```python
from build123d import *

# Parameters (mm, degrees)
SKETCH3_W              = 20
SKETCH3_H              = 50
BOSS_EXTRUDE1_DEPTH    = 35
SKETCH4_R              = 4.75
CUT_EXTRUDE1_DEPTH     = 60
SKETCH5_R              = 3
CUT_EXTRUDE2_DEPTH     = 60
EXTRUDE_2_DEPTH        = 20
SKETCH_3_R             = 2
EXTRUDE_4_DEPTH        = 5
PATTERN_LINEAR_1_COUNT = 2
PATTERN_LINEAR_1_PITCH = 15
SKETCH_5_W             = 20
SKETCH_5_H             = 50
EXTRUDE_5_DEPTH        = 15
SKETCH_6_W             = 4.961104437
SKETCH_6_H             = 10
CUT_EXTRUDE_1_DEPTH    = 10
SKETCH_7_R             = 1.5
CUT_EXTRUDE_2_DEPTH    = 20
SKETCH_8_R             = 4
CUT_EXTRUDE_3_DEPTH    = 20
FILLET_11_R            = 5
FILLET_12_R            = 5
FILLET_START           = -0.209677419
FILLET_13_DEPTH        = 30


with BuildPart() as part:
    # Sketch3 → Boss-Extrude1 (new body)
    with BuildSketch(Plane(origin=(0, 0, 0), x_dir=(1, 0, 0), z_dir=(0, 1, 0))):
        with Locations((-3.806451613, -14.790322581)):
            Rectangle(SKETCH3_W, SKETCH3_H)
    extrude(amount=BOSS_EXTRUDE1_DEPTH)

    # Sketch4 → Cut-Extrude1 (cut)
    with BuildSketch(Plane.XY.offset(39.790322581)):
        with Locations((-3.806451613, 10)):
            Circle(SKETCH4_R)
    extrude(amount=-CUT_EXTRUDE1_DEPTH, mode=Mode.SUBTRACT)

    # Sketch5 → Cut-Extrude2 (cut)
    with BuildSketch(Plane(origin=(6.193548387, 0, 0), x_dir=(0, 0, -1), z_dir=(1, 0, 0))):
        with Locations((-34.790322581, 25)):
            Circle(SKETCH5_R)
        with Locations((5.209677419, 25)):
            Circle(SKETCH5_R)
    extrude(amount=-CUT_EXTRUDE2_DEPTH, mode=Mode.SUBTRACT)

    # 草圖2 → 填料-伸長2 (add)
    with BuildSketch(Plane(origin=(6.193548387, 0, 0), x_dir=(0, 0, -1), z_dir=(1, 0, 0))):
        Polygon((10.209677419, 32.525099494), (10.209677419, 17.525099494), (13.209677419, 22.525099494), (13.209677419, 27.525099494), align=None)
        Polygon((-39.790322581, 17.525099494), (-42.790322581, 22.525099494), (-42.790322581, 27.525099494), (-39.790322581, 32.525099494), align=None)
    extrude(amount=-EXTRUDE_2_DEPTH)

    # 草圖3 → 填料-伸長4 (add)
    # profile 1 of 2: a face of its own
    with BuildSketch(Plane(origin=(6.193548387, 0, 0), x_dir=(0, 0, -1), z_dir=(1, 0, 0))):
        with BuildLine():
            Line((13.209677419, 27.525099494), (17.601982265, 24.989201109))
            ThreePointArc((17.601982265, 24.989201109), (19.46568557, 20.489823314), (15.601982265, 17.525099494))
            Line((15.601982265, 17.525099494), (10.209677419, 17.525099494))
            Line((10.209677419, 17.525099494), (13.209677419, 22.525099494))
            Line((13.209677419, 22.525099494), (13.209677419, 27.525099494))
        make_face()
        with Locations((15.601982265, 21.525099494)):
            Circle(SKETCH_3_R, mode=Mode.SUBTRACT)
    # profile 2 of 2: a face of its own
    with BuildSketch(Plane(origin=(6.193548387, 0, 0), x_dir=(0, 0, -1), z_dir=(1, 0, 0))):
        with BuildLine():
            Line((-39.790322581, 17.525099494), (-45.182627426, 17.525099494))
            ThreePointArc((-45.182627426, 17.525099494), (-49.046330731, 20.489823314), (-47.182627426, 24.989201109))
            Line((-47.182627426, 24.989201109), (-42.790322581, 27.525099494))
            Line((-42.790322581, 27.525099494), (-42.790322581, 22.525099494))
            Line((-42.790322581, 22.525099494), (-39.790322581, 17.525099494))
        make_face()
        with Locations(Location((-45.182627426, 21.525099494, 0), (0, 0, 180))):
            Circle(SKETCH_3_R, mode=Mode.SUBTRACT)
    extrude_4 = extrude(amount=-EXTRUDE_4_DEPTH)

    # 直線複製排列1: 填料-伸長4 ×2
    with Locations(*[(-i * PATTERN_LINEAR_1_PITCH, 0, 0) for i in range(1, PATTERN_LINEAR_1_COUNT)]):
        add(extrude_4)

    # 草圖5 → 填料-伸長5 (add)
    with BuildSketch(Plane(origin=(0, 35, 0), x_dir=(1, 0, 0), z_dir=(0, 1, 0))):
        with Locations((-23.806451613, -14.790322581)):
            Rectangle(SKETCH_5_W, SKETCH_5_H)
    extrude(amount=-EXTRUDE_5_DEPTH)

    # 草圖6 → 除料-伸長1 (cut)
    with BuildSketch(Plane.XZ.offset(-20)):
        with Locations((-16.287003832, -5.209677419)):
            Rectangle(SKETCH_6_W, SKETCH_6_H)
        with Locations((-16.287003832, 34.790322581)):
            Rectangle(SKETCH_6_W, SKETCH_6_H)
    extrude(amount=-CUT_EXTRUDE_1_DEPTH, mode=Mode.SUBTRACT)

    # 草圖7 → 除料-伸長2 (cut)
    with BuildSketch(Plane.ZY.offset(33.806451613)):
        with Locations((-5.209677419, 25)):
            Circle(SKETCH_7_R)
        with Locations((34.790322581, 25)):
            Circle(SKETCH_7_R)
    extrude(amount=-CUT_EXTRUDE_2_DEPTH, mode=Mode.SUBTRACT)

    # 草圖8 → 除料-伸長3 (cut)
    with BuildSketch(Plane(origin=(0, 35, 0), x_dir=(1, 0, 0), z_dir=(0, 1, 0))):
        with Locations(Location((-23.806451613, -15.073492492, 0), (0, 0, 270))):
            Circle(SKETCH_8_R)
    extrude(amount=-CUT_EXTRUDE_3_DEPTH, mode=Mode.SUBTRACT)

    # 圓角11
    fillet_11_edges = [part.edges().sort_by_distance(p)[0] for p in [
        (-26.287003832, 20, -10.209677419),
    ]]
    fillet(fillet_11_edges, radius=FILLET_11_R)

    # 圓角12
    fillet_12_edges = [part.edges().sort_by_distance(p)[0] for p in [
        (-26.287003832, 20, 39.790322581),
    ]]
    fillet(fillet_12_edges, radius=FILLET_12_R)

    # 圓角13: read off the stored shape, not the designer's step
    # 圓角13 outline → 圓角13 (add)
    with BuildSketch(Plane.XY.offset(FILLET_START)):
        with BuildLine():
            Line((-13.806451613, 20), (-17.341985519, 20))
            ThreePointArc((-17.341985519, 20), (-14.841985519, 18.964466094), (-13.806451613, 16.464466094))
            Line((-13.806451613, 16.464466094), (-13.806451613, 20))
        make_face()
    extrude(amount=FILLET_13_DEPTH)


solid = part.part
```
Verification items for the finished model (mm, model axes). A direction names the side the tool comes from. Give positions to 0.01 mm unless a question says otherwise; leave off trailing zeros. Loops run counter-clockwise (first coordinate to the right, second up) from the corner with the lowest first, then second, coordinate; pieces in that order, holes last. Notation, with made-up numbers: M 4.5,81.25 L 45.5,81.25 A12 ccw 45.5,89.25 Z; hole C 12.5,64 d5. An arc over 180 degrees is marked long. Return JSON: item names as keys, results as strings.
1) Section check D-D, the plane z = 26. Enter the section's corners in (x, y), and give its area (3 significant figures).
Findings:
{"outline": "M -33.81,20 L -17.34,20 A3.54 cw -13.81,16.46 L -13.81,0 L 6.19,0 L 6.19,35 L -33.81,35 Z; hole C -3.81,10 d9.5", "area": "932 mm2"}
2) Mould release check, pull along Y, two halves, no side actions. Record for faces 4 (the cylindrical face through (3.729, 20.561, -19.484)), 5 (the flat face through (-3.67, 29.99, 41.31)), 6 (the cylindrical face through (-11.27, 22.29, 47.03)), 7 (the cylindrical face through (-26.18, 21.43, 38.29)): released by +Y, released by -Y, zero draft, split by the parting line, or undercut.
Findings:
{"face 4": "split by the parting line", "face 5": "released by +Y", "face 6": "undercut", "face 7": "released by -Y"}
3) Material ranges on L1, parallel to X at y = 27.5, z = 36.5; L2, parallel to Y at x = 1, z = 35; L3, parallel to Y at x = -4.5, z = 37.5, recorded low to high. Write a range as [from, to].
Findings:
{"L1": "x = [-33.81, -18.77], [-13.81, 6.19]", "L2": "y = [0, 22.01], [27.99, 35]", "L3": "y = [0, 5.3], [14.7, 23.71], [26.29, 35]"}
4) Section check C-C, the plane x = -22.5. Enter the section's corners in (y, z).
Findings:
{"outline": "M 20,-5.21 A5 ccw 25,-10.21 L 35,-10.21 L 35,11.29 L 20,11.29 Z; M 20,18.85 L 35,18.85 L 35,39.79 L 25,39.79 A5 ccw 20,34.79 Z; hole C 25,-5.21 d3; hole C 25,34.79 d3"}
5) Gauge pin test, flat ends, axial feed: P1, Ø3, axis at y = 20.5, z = 41, coming from the -X side; P2, Ø5, axis at x = -28, z = 16.5, coming from the -Y side; P3, Ø2, axis at x = -22, y = 27, coming from the +Z side. Record the tip position at first contact, or that the pin passes through.
Findings:
{"P1": "stops at x = -13.81", "P2": "stops at y = 20", "P3": "stops at z = 39.79"}
6) Tool access check on faces 1 (the flat face through (-19, 31, -10.21)), 2 (the flat face through (-4, 5, -10.21)), 3 (the flat face through (1.194, 20, -14)). Record the directions out of +Z, -Z, +X, -X, +Y, -Y that give a thin tool (end or side, any length) a straight path to the whole face; none if there is none.
Findings:
{"face 1": "-Z, -X, +Y", "face 2": "-Z, +X, -X, -Y", "face 3": "-Z, -Y"}
7) Section check A-A, the plane y = 10. Enter the section's corners in (x, z).
Findings:
{"outline": "M -13.81,-10.21 L -8.56,-10.21 L -8.56,39.79 L -13.81,39.79 Z; M 0.94,-10.21 L 6.19,-10.21 L 6.19,39.79 L 0.94,39.79 Z"}
8) Section check B-B, the plane z = 18. Enter the section's corners in (x, y).
Findings:
{"outline": "M -33.81,20 L -26.53,20 L -26.53,35 L -33.81,35 Z; M -21.08,20 L -17.34,20 A3.54 cw -13.81,16.46 L -13.81,0 L 6.19,0 L 6.19,35 L -21.08,35 Z; hole C -3.81,10 d9.5"}
